Source: CAD feature listing. Evaluate the final solid. Frame: model axes, mm. Give positions to 0.01 mm unless a question says otherwise; leave off trailing zeros. Loops run counter-clockwise (first coordinate to the right, second up) from the corner with the lowest first, then second, coordinate; pieces in that order, holes last. Notation, with made-up numbers: M -31.5,35 L 24.5,35 A13 ccw 24.5,43 Z; hole C -24.75,-20.75 d8. An arc over 180 degrees is marked long. Put each result on its own line as item: value.
from build123d import *

# Parameters (mm, degrees)
SKETCH_1_W                  = 1060
SKETCH_1_H                  = 610
EXTRUDE_1_DEPTH             = 10
CUT_EXTRUDE_2_DEPTH         = 10
HOLE_WIZARD_16_0_16_1_D     = 16
HOLE_WIZARD_16_0_16_1_DEPTH = 42
HOLE_WIZARD_16_0_16_1_TIP   = 4.806884952
SKETCH_6_R                  = 40
SKETCH_6_R_2                = 60
SKETCH_6_R_3                = 90
CUT_EXTRUDE_3_DEPTH         = 1224.029026638


with BuildPart() as part:
    # 草图1 → 凸台-拉伸1 (new body)
    with BuildSketch(Plane.XY):
        with Locations((530, 305)):
            Rectangle(SKETCH_1_W, SKETCH_1_H)
    extrude(amount=EXTRUDE_1_DEPTH)

    # 草图3 → 切除-拉伸2 (cut)
    with BuildSketch(Plane.XY.offset(10)):
        Polygon((0, 305), (300, 0), (0, 0), align=None)
        Polygon((1060, 305), (760, 0), (1060, 0), align=None)
        with BuildLine():
            Line((935.312302429, 610), (124.687697571, 610))
            ThreePointArc((124.687697571, 610), (530, 334.25), (935.312302429, 610))
        make_face()
    extrude(amount=-CUT_EXTRUDE_2_DEPTH, mode=Mode.SUBTRACT)

    # Ø16.0 (16) 直径孔1
    with Locations(Plane(origin=(0, 0, 0), x_dir=(-1, 0, 0), z_dir=(0, 0, -1))):
        with Locations((-1030, 580), (-1030, 360), (-730, 30), (-330, 30), (-30, 360), (-30, 580), (-680, 260), (-380, 260)):
            Hole(HOLE_WIZARD_16_0_16_1_D / 2, depth=HOLE_WIZARD_16_0_16_1_DEPTH)
            with Locations((0, 0, -(HOLE_WIZARD_16_0_16_1_DEPTH + HOLE_WIZARD_16_0_16_1_TIP / 2))):  # 118° drill point
                Cone(0, HOLE_WIZARD_16_0_16_1_D / 2, HOLE_WIZARD_16_0_16_1_TIP, mode=Mode.SUBTRACT)

    # 草图6 → 切除-拉伸3 (cut, through all)
    with BuildSketch(Plane(origin=(0, 0, 0), x_dir=(-1, 0, 0), z_dir=(0, 0, -1))):
        with Locations((-970, 460)):
            Circle(SKETCH_6_R)
        with Locations((-850, 280)):
            Circle(SKETCH_6_R_2)
        with Locations((-530, 160)):
            Circle(SKETCH_6_R_3)
        with Locations((-210, 280)):
            Circle(SKETCH_6_R_2)
        with Locations((-90, 460)):
            Circle(SKETCH_6_R)
    extrude(amount=-CUT_EXTRUDE_3_DEPTH, mode=Mode.SUBTRACT)


solid = part.part
1. Contact query for flat-ended pins moving along their axis: P1, Ø3, axis at y = 130.5, z = 4.5, coming from the -X side; P2, Ø3, axis at x = 192.5, z = 2.5, coming from the -Y side; P3, Ø4, axis at y = 226, z = 4, coming from the -X side. Output: stop coordinate, or through.
Found:
P1: x = 170.16
P2: y = 107.77
P3: x = 75.74
2. Draft query along X for faces 1 (the cylindrical face through (522.71, 334.31, 5.07)), 2 (the flat face through (912.1, 154.635, 5.07)), 3 (the flat face through (523, 309, 10)). Return one class per face: pulls with the +X half, pulls with the -X half, needs draft (parallel to the pull), parting line crosses it, or undercut.
Found:
face 1: undercut
face 2: pulls with the +X half
face 3: needs draft
3. Section query B-B (y = 88). Output: boundary loops of the cut face in (x, z), plus the area to 3 significant figures.
Found:
outline: M 213.44,0 L 476,0 L 476,10 L 213.44,10 Z; M 584,0 L 846.56,0 L 846.56,10 L 584,10 Z
area: 5,250 mm^2
4. Section query C-C (y = 280). Output: boundary loops of the cut face in (x, z).
Found:
outline: M 24.59,0 L 150,0 L 150,10 L 24.59,10 Z; M 270,0 L 790,0 L 790,10 L 270,10 Z; M 910,0 L 1035.41,0 L 1035.41,10 L 910,10 Z
5. Section query A-A (x = 970). Output: boundary loops of the cut face in (y, z).
Found:
outline: M 213.5,0 L 420,0 L 420,10 L 213.5,10 Z; M 500,0 L 610,0 L 610,10 L 500,10 Z
6. Material intervals for line 1 (X direction, y = 439, z = 3.25); line 2 (X direction, y = 580, z = 4.75); line 3 (X direction, y = 250.5, z = 5.25), sorted ascending. Write a range as from..to.
Found:
line 1: 0..55.96, 124.04..246.6, 813.4..935.96, 1004.04..1060
line 2: 0..22, 38..137.85, 922.15..1022, 1038..1060
line 3: 53.61..157.75, 262.25..797.75, 902.25..1006.39
7. Section query D-D (z = 5.5). State how many separate pieces and enclosed holes the cut face has, plus the area to 3 significant figures.
Found:
separate pieces: 1
enclosed holes: 13
area: 333,000 mm^2
